Verification items for the finished model (mm, model axes). Face numbers are marked on the shaded views. A direction names the side the tool comes from. Coordinates: 2 decimals unless noted, no trailing zeros. Write each loop counter-clockwise with the first axis right and the second up, starting at its lowest first coordinate (ties: lowest second). Pieces come first, ordered by that corner, then holes. Notation, with made-up numbers: (61, 80.5) -> (110, 80.5) arc R8 cw to (110, 86.5) -> close; hole circle Ø5 at (77, 63). An arc over 180 degrees is marked (long way). Answer in a Markdown table with one row per item.
```python
from build123d import *

# Parameters (mm, degrees)
SKETCH1_W           = 6.2
SKETCH1_H           = 10.2
BOSS_EXTRUDE1_DEPTH = 2
SKETCH3_W           = 0.2
SKETCH3_H           = 0.05
BOSS_EXTRUDE3_DEPTH = 10
CUT_EXTRUDE1_DEPTH  = 0.05
BOSS_EXTRUDE4_DEPTH = 7.2


with BuildPart() as part:
    # Sketch1 → Boss-Extrude1 (new body)
    with BuildSketch(Plane(origin=(0, 0, 0), x_dir=(1, 0, 0), z_dir=(0, 1, 0))):
        Polygon((-3.6, -6.1), (-3.1, -6.1), (3.1, -6.1), (3.6, -6.1), (3.6, 6.1), (-3.6, 6.1), align=None)
        with Locations((0, -11.2)):
            Rectangle(SKETCH1_W, SKETCH1_H)
    extrude(amount=BOSS_EXTRUDE1_DEPTH)

    # Sketch3 → Boss-Extrude3 (add)
    with BuildSketch(Plane.XY.offset(16.3)):
        with Locations((0, 1)):
            Rectangle(SKETCH3_W, SKETCH3_H)
    extrude(amount=BOSS_EXTRUDE3_DEPTH)

    # Sketch4 → Cut-Extrude1 (cut)
    with BuildSketch(Plane.XZ.offset(-0.975)):
        Polygon((0.1, 26.3), (0, 26.3), (0.1, 26), align=None)
        Polygon((-0.1, 26.3), (-0.1, 26), (0, 26.3), align=None)
    extrude(amount=-CUT_EXTRUDE1_DEPTH, mode=Mode.SUBTRACT)

    # Sketch5 → Boss-Extrude4 (add)
    with BuildSketch(Plane(origin=(3.6, 0, 0), x_dir=(0, 0, -1), z_dir=(1, 0, 0))):
        with BuildLine():
            Line((6.1, 1.261801628), (6.1, 0.942348221))
            add(Edge.make_bspline(
                [(6.1, 0.942348221), (24.518318323, 0.810344541), (46.52588684, -0.554134336)],
                knots=[0, 0, 0, 1, 1, 1], degree=2))
            Line((46.52588684, -0.554134336), (46.52588684, -0.234680929))
            add(Edge.make_bspline(
                [(6.1, 1.261801628), (24.562430755, 1.083380731), (46.52588684, -0.234680929)],
                knots=[0, 0, 0, 1, 1, 1], degree=2))
        make_face()
    extrude(amount=-BOSS_EXTRUDE4_DEPTH)


solid = part.part
```
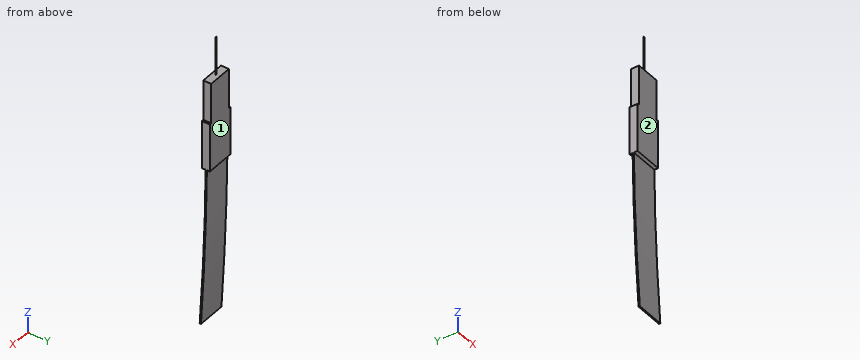
1. Access from +Z, -Z, +X, -X, +Y, -Y to the whole of each face (thin tool, end or side, straight path). Record for the marked faces 1 and 2.
Findings below:
| item | result |
|---|---|
| face 1 | +Z, -Z, +X, -X, +Y |
| face 2 | +Z, +X, -X, -Y |
2. Sectioned sample at A-A, the plane z = -1.5. Record the cut outline in (x, y).
Findings below:
| item | result |
|---|---|
| outline | (-3.6, 0) -> (3.6, 0) -> (3.6, 2) -> (-3.6, 2) -> close |
3. Sectioned sample at B-B, the plane z = 7. Record the cut outline in (x, y), and give its area (3 significant figures).
Findings below:
| item | result |
|---|---|
| outline | (-3.1, 0) -> (3.1, 0) -> (3.1, 2) -> (-3.1, 2) -> close |
| area | 12.4 mm² |
4. Go/stop test with flat-tipped pins: pin 1 (1.5 mm diameter, centred on y = 1.5, z = -14, fed in from +X); pin 2 (0.6 mm diameter, centred on x = 0.5, y = 1, fed in from +Z); pin 3 (0.6 mm diameter, centred on y = 1, z = 9.5, fed in from +X); pin 4 (1 mm diameter, centred on x = -1.5, z = -31.5, fed in from +Y). Record where each tip stops, or that it passes through.
Findings below:
| item | result |
|---|---|
| pin 1 | stops at x = 3.6 |
| pin 2 | stops at z = 16.3 |
| pin 3 | stops at x = 3.1 |
| pin 4 | stops at y = 0.57 |
5. Material ranges on probe 1 along Z at (x, y) = (1, 1.45); probe 2 along Y at (x, z) = (3, 3.5); probe 3 along X at (y, z) = (1.2, 9), recorded low to high. Write a range as from..to.
Findings below:
| item | result |
|---|---|
| probe 1 | z = -6.1..16.3 |
| probe 2 | y = 0..2 |
| probe 3 | x = -3.1..3.1 |
